Source: CAD feature listing. Evaluate the final solid. Frame: model axes, mm. A direction names the side the tool comes from. Coordinates: 2 decimals unless noted, no trailing zeros. Write each loop counter-clockwise with the first axis right and the second up, starting at its lowest first coordinate (ties: lowest second). Pieces come first, ordered by that corner, then holes. Notation, with made-up numbers: (-29, 6) -> (22, 6) arc R14 cw to (22, 16) -> close; hole circle Ø5 at (36, 1.25). An arc over 180 degrees is marked (long way). One line per item, written item: value. Start each with the question number.
1. Access query for faces 1 (the cylindrical face through (-23.55, -7.01, -1.97)), 2 (the flat face through (-12, -26, 7)), 3 (the flat face through (-21.514, -7.474, 10.07)), 4 (the flat face through (-21, -13.5, 6)), 5 (the flat face through (-21, -19, 14)). Directions: +Z, -Z, +X, -X, +Y, -Y. A direction counts if a zero-diameter tool reaches every point of the face in a straight line with its end or side. Return the directions, or none.
2. Section query B-B, the plane y = -16.5. Output: boundary loops of the cut face in (x, z).
3. Section query C-C, the plane x = -15.5. Output: boundary loops of the cut face in (y, z).
4. Section query D-D, the plane z = 12.25. Output: boundary loops of the cut face in (x, y), and give its area (3 significant figures).
5. Section query A-A, the plane z = 7.5. Output: boundary loops of the cut face in (x, y).
6. Mould query, pull axis Y, two halves, no side actions, for faces 6 (the flat face through (-22.5, -6, 10)), 7 (the flat face through (0, 2.5, 7)), 8 (the flat face through (-22, -47.5, 14)), 9 (the flat face through (-21, -46, 13)). Classes: released by +Y, released by -Y, zero draft, split by the parting line, or undercut.
7. First-contact query: P1, Ø4.5, axis at x = -20, y = -6.5, coming from the +Z side; P2, Ø4, axis at x = -18.5, z = 3.5, coming from the -Y side; P3, Ø5, axis at y = -41.5, z = 5.5, coming from the +X side; P4, Ø4.5, axis at x = -20, y = -43.5, coming from the -Z side. Flat tips, straight axial feed; report the tip coordinate or a pass-through.
8. Line query: line 1 (Y direction, x = -20.5, z = 14.5); line 2 (Y direction, x = -20.5, z = 0.25); line 3 (Z direction, x = 25, y = 0). Output: solid intervals per line, ascending.
from build123d import *

# Parameters (mm, degrees)
DODANIE_WYCI_GNI_CIE1_DEPTH = 15
OTW_R_POD_RUB_M21_D         = 2.6
OTW_R_POD_RUB_M21_DEPTH     = 5
SZKIC7_W                    = 13
SZKIC7_H                    = 34
WYTNIJ_WYCI_GNI_CIE2_DEPTH  = 13
WYTNIJ_WYCI_GNI_CIE3_REACH  = 4
SZKIC8_W                    = 13
SZKIC8_H                    = 23
OTW_R_POD_RUB_M22_D         = 2.6
OTW_R_POD_RUB_M22_DEPTH     = 2
SZKIC13_R                   = 3.3
DODANIE_WYCI_GNI_CIE2_DEPTH = 4
WYTNIJ_WYCI_GNI_CIE4_REACH  = 21
SZKIC11_R                   = 1.3
WYTNIJ_WYCI_GNI_CIE5_DEPTH  = 10
ZAOKR_GLENIE1_R             = 3


with BuildPart() as part:
    # Szkic1 → Dodanie-wyciągnięcie1 (new body)
    with BuildSketch(Plane.XY):
        Polygon((-30, -2.5), (-30, 2.5), (30, 2.5), (30, -2.5), (-12, -2.5), (-12, -47.5), (-30, -47.5), align=None)
    extrude(amount=DODANIE_WYCI_GNI_CIE1_DEPTH)

    # Otwór pod śrubę M21
    with Locations(Plane(origin=(0, 2.5, 0), x_dir=(-1, 0, 0), z_dir=(0, 1, 0))):
        with Locations((-25, 7.5), (4, 7.5)):
            Hole(OTW_R_POD_RUB_M21_D / 2, depth=OTW_R_POD_RUB_M21_DEPTH)

    # Szkic7 → Wytnij-wyciągnięcie2 (cut)
    with BuildSketch(Plane(origin=(0, 0, 0), x_dir=(-1, 0, 0), z_dir=(0, 0, -1))):
        with Locations((21, -30.5)):
            Rectangle(SZKIC7_W, SZKIC7_H)
    extrude(amount=-WYTNIJ_WYCI_GNI_CIE2_DEPTH, mode=Mode.SUBTRACT)

    # Szkic8 → Wytnij-wyciągnięcie3 (cut, up to next)
    with BuildSketch(Plane(origin=(0, 0, 13), x_dir=(-1, 0, 0), z_dir=(0, 0, -1)), mode=Mode.PRIVATE) as wytnij_wyci_gni_cie3_sk1:
        with Locations((21, -30.5)):
            Rectangle(SZKIC8_W, SZKIC8_H)
    wytnij_wyci_gni_cie3_tool1 = extrude(wytnij_wyci_gni_cie3_sk1.sketch, amount=-WYTNIJ_WYCI_GNI_CIE3_REACH, mode=Mode.PRIVATE) & part.part
    add(wytnij_wyci_gni_cie3_tool1.solids().sort_by_distance((-21, -30.5, 13))[0], mode=Mode.SUBTRACT)

    # Otwór pod śrubę M22
    with Locations(Plane(origin=(0, 0, 13), x_dir=(-1, 0, 0), z_dir=(0, 0, -1))):
        with Locations((20.5, -16.5), (20.5, -44.5)):
            Hole(OTW_R_POD_RUB_M22_D / 2, depth=OTW_R_POD_RUB_M22_DEPTH)

    # Szkic13 → Dodanie-wyciągnięcie2 (add)
    with BuildSketch(Plane(origin=(0, 0, 0), x_dir=(-1, 0, 0), z_dir=(0, 0, -1))):
        with Locations((20.5, -5.75)):
            Circle(SZKIC13_R)
    extrude(amount=DODANIE_WYCI_GNI_CIE2_DEPTH)

    # Szkic11 → Wytnij-wyciągnięcie4 (cut, up to next)
    with BuildSketch(Plane(origin=(0, 0, -4), x_dir=(-1, 0, 0), z_dir=(0, 0, -1)), mode=Mode.PRIVATE) as wytnij_wyci_gni_cie4_sk1:
        with Locations((20.5, -5.75)):
            Circle(SZKIC11_R)
    wytnij_wyci_gni_cie4_tool1 = extrude(wytnij_wyci_gni_cie4_sk1.sketch, amount=-WYTNIJ_WYCI_GNI_CIE4_REACH, mode=Mode.PRIVATE) & part.part
    add(wytnij_wyci_gni_cie4_tool1.solids().sort_by_distance((-20.5, -5.75, -4))[0], mode=Mode.SUBTRACT)

    # Szkic12 → Wytnij-wyciągnięcie5 (cut)
    with BuildSketch(Plane.XY.offset(15)):
        Polygon((-18.5, -6.904700538), (-18.5, -4.595299462), (-20.5, -3.440598923), (-22.5, -4.595299462), (-22.5, -6.904700538), (-20.5, -8.059401077), align=None)
    extrude(amount=-WYTNIJ_WYCI_GNI_CIE5_DEPTH, mode=Mode.SUBTRACT)

    # Zaokrąglenie1
    zaokr_glenie1_edges = [part.edges().sort_by_distance(p)[0] for p in [
        (-12, -2.5, 7.5),
    ]]
    fillet(zaokr_glenie1_edges, radius=ZAOKR_GLENIE1_R)


solid = part.part
Computed values:
1. face 1: -Z
1. face 2: +Z, -Z, +X, -Y
1. face 3: +Z
1. face 4: -Z, -Y
1. face 5: +Z, -Z
2. outline: (-30, 0) -> (-27.5, 0) -> (-27.5, 13) -> (-21.8, 13) -> (-21.8, 15) -> (-30, 15) -> close; (-19.2, 13) -> (-14.5, 13) -> (-14.5, 0) -> (-12, 0) -> (-12, 15) -> (-19.2, 15) -> close
3. outline: (-47.5, 13) -> (-42, 13) -> (-42, 15) -> (-47.5, 15) -> close; (-19, 13) -> (-13.5, 13) -> (-13.5, 0) -> (2.5, 0) -> (2.5, 15) -> (-19, 15) -> close
4. outline: (-30, -47.5) -> (-27.5, -47.5) -> (-27.5, -13.5) -> (-14.5, -13.5) -> (-14.5, -47.5) -> (-12, -47.5) -> (-12, -5.5) arc R3 cw to (-9, -2.5) -> (30, -2.5) -> (30, 2.5) -> (-30, 2.5) -> close; hole (-22.5, -6.9) -> (-20.5, -8.06) -> (-18.5, -6.9) -> (-18.5, -4.6) -> (-20.5, -3.44) -> (-22.5, -4.6) -> close
4. area: 656 mm²
5. outline: (-30, -47.5) -> (-27.5, -47.5) -> (-27.5, -13.5) -> (-14.5, -13.5) -> (-14.5, -47.5) -> (-12, -47.5) -> (-12, -5.5) arc R3 cw to (-9, -2.5) -> (-5.3, -2.5) -> (-5.3, 2.5) -> (-30, 2.5) -> close; (-2.7, -2.5) -> (23.7, -2.5) -> (23.7, 2.5) -> (-2.7, 2.5) -> close; (26.3, -2.5) -> (30, -2.5) -> (30, 2.5) -> (26.3, 2.5) -> close; hole (-22.5, -6.9) -> (-20.5, -8.06) -> (-18.5, -6.9) -> (-18.5, -4.6) -> (-20.5, -3.44) -> (-22.5, -4.6) -> close
6. face 6: undercut
6. face 7: released by +Y
6. face 8: released by -Y
6. face 9: zero draft
7. P1: stops at z = 15
7. P2: stops at y = -13.5
7. P3: stops at x = -12
7. P4: stops at z = 13
8. line 1: y = -47.5 to -45.8, -43.2 to -42, -19 to -17.8, -15.2 to -8.06, -3.44 to 2.5
8. line 2: y = -13.5 to -7.05, -4.45 to 2.5
8. line 3: z = 0 to 6.2, 8.8 to 15
